Geometry: final body of the model. Coordinates: model frame, mm. Face numbers are marked on the shaded views. A direction names the side the tool comes from. Give positions to 0.01 mm unless a question says otherwise; leave off trailing zeros. Write each loop counter-clockwise with the first axis right and the second up, starting at its lowest first coordinate (ties: lowest second). Pieces come first, ordered by that corner, then holes. Notation, with made-up numbers: M 29.5,58 L 67.5,58 A16 cw 67.5,71 Z; hole C 46.5,13.25 d5. An arc over 180 degrees is marked long. Use one line per item in the form item = value. Start each with the question number.
Item 1: Pull-direction query (X, two-part tool) for the marked faces 1, 2, 3 and 4; classes: released by +X, released by -X, zero draft, split by the parting line, or undercut.
Item 2: Section query B-B on y = 0. Return loops of the section in (x, z).
Item 3: Contact query for flat-ended pins moving along their axis: P1, Ø8, axis at x = 4.5, z = 16, coming from the +Y side; P2, Ø3, axis at x = -2.5, z = 11.5, coming from the -Y side; P3, Ø1.5, axis at y = 3.5, z = 4.5, coming from the +X side. Output: stop coordinate, or through.
Item 4: Section query C-C on x = 18.75. Return loops of the section in (y, z), then the cut area to 3 significant figures.
Item 5: Section query D-D on z = 7.5. Return loops of the section in (x, y).
Item 6: Access query for the marked faces 5 and 6. Directions: +Z, -Z, +X, -X, +Y, -Y. A direction counts if a zero-diameter tool reaches every point of the face in a straight line with its end or side. Return the directions, or none.
Item 7: Section query A-A on z = 15.25. Return loops of the section in (x, y), then the cut area to 3 significant figures.
Item 8: Material intervals for line 1 along Y through (x, z) = (0, 17); line 2 along X through (y, z) = (-2.5, 17.25); line 3 along Z through (x, y) = (4, -3.5), sorted ascending. Write a range as from..to.
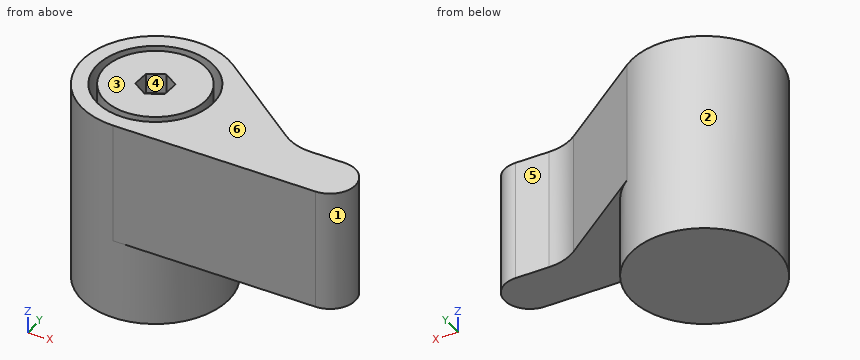
from build123d import *

# Parameters (mm, degrees)
SKETCH_1_R          = 7.25
EXTRUDE_1_DEPTH     = 20
EXTRUDE_2_DEPTH     = 12
FILLET_1_R          = 5
SKETCH_3_R          = 5.75
CUT_EXTRUDE_1_DEPTH = 10
SKETCH_4_R          = 5
EXTRUDE_3_DEPTH     = 10
CUT_EXTRUDE_2_DEPTH = 2


with BuildPart() as part:
    # Эскиз1 → Бобышка-Вытянуть1 (new body)
    with BuildSketch(Plane.XY):
        Circle(SKETCH_1_R)
    extrude(amount=EXTRUDE_1_DEPTH)

    # Эскиз2 → Бобышка-Вытянуть2 (add)
    with BuildSketch(Plane.XY.offset(20)):
        with BuildLine():
            Line((0, -7.25), (20, -7.25))
            ThreePointArc((20, -7.25), (22.5, -4.75), (20, -2.25))
            Line((20, -2.25), (15, -2.25))
            Line((15, -2.25), (4.371714259, 5.783650615))
            ThreePointArc((4.371714259, 5.783650615), (-6.873644119, 2.305540397), (0, -7.25))
        make_face()
    extrude(amount=-EXTRUDE_2_DEPTH)

    # Скругление1
    fillet_1_edges = [part.edges().sort_by_distance(p)[0] for p in [
        (15, -2.25, 14),
    ]]
    fillet(fillet_1_edges, radius=FILLET_1_R)

    # Эскиз3 → Вырез-Вытянуть1 (cut)
    with BuildSketch(Plane.XY.offset(20)):
        Circle(SKETCH_3_R)
    extrude(amount=-CUT_EXTRUDE_1_DEPTH, mode=Mode.SUBTRACT)

    # Эскиз4 → Бобышка-Вытянуть3 (add)
    with BuildSketch(Plane.XY.offset(10)):
        Circle(SKETCH_4_R)
    extrude(amount=EXTRUDE_3_DEPTH)

    # Эскиз5 → Вырез-Вытянуть2 (cut)
    with BuildSketch(Plane.XY.offset(20)):
        Polygon((1.457985788, -0.935028044), (1.538750933, 0.795138708), (0.080765145, 1.730166752), (-1.457985788, 0.935028044), (-1.538750933, -0.795138708), (-0.080765145, -1.730166752), align=None)
    extrude(amount=-CUT_EXTRUDE_2_DEPTH, mode=Mode.SUBTRACT)


solid = part.part
Answer sheet:
q1.face_1 = released by +X
q1.face_2 = split by the parting line
q1.face_3 = zero draft
q1.face_4 = undercut
q2.outline = M -7.25,0 L 7.25,0 L 7.25,8 L 12.02,8 L 12.02,20 L 5.75,20 L 5.75,10 L 5,10 L 5,20 L 1.5,20 L 1.5,18 L -1.5,18 L -1.5,20 L -5,20 L -5,10 L -5.75,10 L -5.75,20 L -7.25,20 Z
q3.P1 = 7.23
q3.P2 = -7.18
q3.P3 = 6.71
q4.outline = M -7.25,8 L -2.25,8 L -2.25,20 L -7.25,20 Z
q4.area = 60.0 mm2
q5.outline = C 0,0 d14.5
q6.face_5 = +Z, -Z, +X, +Y
q6.face_6 = +Z, +X, -X, +Y, -Y
q7.outline = C 0,0 d10; M 0,-7.25 L 20,-7.25 A2.5 ccw 20,-2.25 L 16.68,-2.25 A5 cw 13.66,-1.24 L 4.37,5.78 A7.25 ccw long Z; hole C 0,0 d11.5
q7.area = 250 mm2
q8.line_1 = -7.25..-5.75, -5..5, 5.75..7.25
q8.line_2 = -6.81..-5.18, -4.33..4.33, 5.18..21.09
q8.line_3 = 0..10
